Read the model definition and answer for the solid it produces. Units are mm, in the model's axes. Give positions to 0.01 mm unless a question says otherwise; leave off trailing zeros. Loops run counter-clockwise (first coordinate to the right, second up) from the corner with the lowest first, then second, coordinate; pieces in that order, holes last. Notation, with made-up numbers: (-2, 78.25) - (23, 78.25) arc R20 ccw to (23, 113.25) - close; hole circle Ø9 at (-29.5, -19). An arc over 180 degrees is marked (long way). Use a Markdown table: item, result. Add a question column.
Item 1: A cutting plane is placed at A-A (x = 12). Determine the outline of the cut face in (y, z), plus the area to 3 significant figures.
Item 2: A cutting plane is placed at B-B (z = -19). Determine the outline of the cut face in (x, y).
Item 3: A cutting plane is placed at C-C (y = 1.5). Determine the outline of the cut face in (x, z).
Item 4: A cutting plane is placed at D-D (x = 29). Determine the outline of the cut face in (y, z), plus the area to 3 significant figures.
Item 5: Each of these flat-tipped pins is pushed along its axis until it touches: P1, Ø3, axis at x = -19.5, y = 2, coming from the +Z side; P2, Ø1.5, axis at x = -29.5, z = 3.5, coming from the -Y side. Where does it stop, or does it pass through?
Item 6: Consider probe 1 along X at (y, z) = (6, 1.5); probe 2 along Z at (x, y) = (-10, 3.25); probe 3 along Z at (x, y) = (38.5, 1.5). Determine where each line is inside the solid, lowest interval first. Write a range as [from, to].
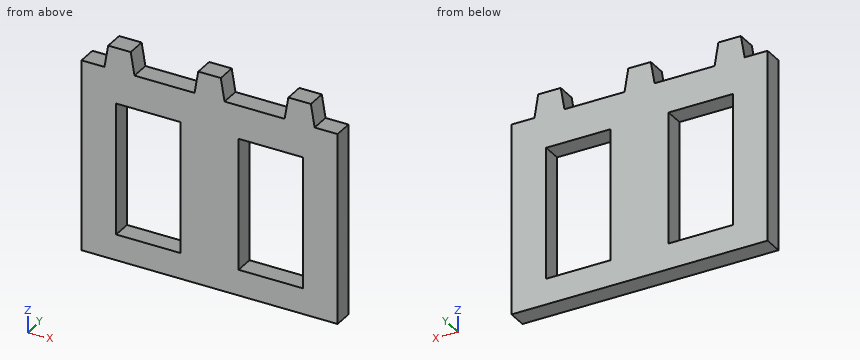
from build123d import *

# Parameters (mm, degrees)
SKETCH2_W           = 85.279590556
SKETCH2_H           = 63.5
SKETCH2_W_2         = 21.432451429
SKETCH2_H_2         = 43.79853014
BOSS_EXTRUDE1_DEPTH = 6.35


with BuildPart() as part:
    # Sketch2 → Boss-Extrude1 (new body)
    with BuildSketch(Plane(origin=(0, 0, 0), x_dir=(1, 0, 0), z_dir=(0, 1, 0))):
        Rectangle(SKETCH2_W, SKETCH2_H)
        with Locations((-20.38588495, 1.25966445)):
            Rectangle(SKETCH2_W_2, SKETCH2_H_2, mode=Mode.SUBTRACT)
        with Locations((20.38588495, 1.25966445)):
            Rectangle(SKETCH2_W_2, SKETCH2_H_2, mode=Mode.SUBTRACT)
        Polygon((-25, -31.75), (-35, -31.75), (-33.75, -39.25), (-26.25, -39.25), align=None)
        Polygon((5, -31.75), (-5, -31.75), (-3.75, -39.25), (3.75, -39.25), align=None)
        Polygon((33.75, -39.25), (35, -31.75), (25, -31.75), (26.25, -39.25), align=None)
    extrude(amount=BOSS_EXTRUDE1_DEPTH)


solid = part.part
Geometry says:
| question | item | result |
|---|---|---|
| 1 | outline | (0, -31.75) - (6.35, -31.75) - (6.35, -23.16) - (0, -23.16) - close; (0, 20.64) - (6.35, 20.64) - (6.35, 31.75) - (0, 31.75) - close |
| 1 | area | 125 mm² |
| 2 | outline | (-42.64, 0) - (-31.1, 0) - (-31.1, 6.35) - (-42.64, 6.35) - close; (-9.67, 0) - (9.67, 0) - (9.67, 6.35) - (-9.67, 6.35) - close; (31.1, 0) - (42.64, 0) - (42.64, 6.35) - (31.1, 6.35) - close |
| 3 | outline | (-42.64, -31.75) - (42.64, -31.75) - (42.64, 31.75) - (35, 31.75) - (33.75, 39.25) - (26.25, 39.25) - (25, 31.75) - (5, 31.75) - (3.75, 39.25) - (-3.75, 39.25) - (-5, 31.75) - (-25, 31.75) - (-26.25, 39.25) - (-33.75, 39.25) - (-35, 31.75) - (-42.64, 31.75) - close; hole (-31.1, -23.16) - (-9.67, -23.16) - (-9.67, 20.64) - (-31.1, 20.64) - close; hole (9.67, -23.16) - (31.1, -23.16) - (31.1, 20.64) - (9.67, 20.64) - close |
| 4 | outline | (0, -31.75) - (6.35, -31.75) - (6.35, -23.16) - (0, -23.16) - close; (0, 20.64) - (6.35, 20.64) - (6.35, 39.25) - (0, 39.25) - close |
| 4 | area | 173 mm² |
| 5 | P1 | z = 31.75 |
| 5 | P2 | through |
| 6 | probe 1 | [-42.64, -31.1], [-9.67, 9.67], [31.1, 42.64] |
| 6 | probe 2 | [-31.75, -23.16], [20.64, 31.75] |
| 6 | probe 3 | [-31.75, 31.75] |
